Could you check a few things on this model? Use its own coordinates, in mm. Face numbers are marked on the shaded views. A direction names the side the tool comes from. Give positions to 0.01 mm unless a question says otherwise; leave off trailing zeros. Order: outer loops, then holes, each group sorted by start corner. A loop starts at its lowest first (then second) coordinate and runs counter-clockwise, first axis right, second up. Notation, with made-up numbers: (79.5, 75) - (134.5, 75) arc R15 ccw to (134.5, 93) - close; hole circle Ø7 at (-35.5, 80.5). An arc over 180 degrees is marked (long way). One line per question, with ' | ' between items. Start each with the question number.
1. Imagine slicing it at A-A (x = 38). Please give me the cut outline in (y, z), and give its area (3 significant figures).
2. Imagine slicing it at C-C (y = 0). Please give me the cut outline in (x, z), and give its area (3 significant figures).
3. Imagine slicing it at B-B (y = 20.5). Please give me the cut outline in (x, z).
4. Which directions (+Z, -Z, +X, -X, +Y, -Y) give clear straight access to the entire face, cutting with the end or side of a thin tool? Please do the marked faces 3 and 4.
5. Imagine slicing it at D-D (z = 12). Please give me the cut outline in (x, y), and give its area (3 significant figures).
6. If we mould it in two halves opening along Y, with no side actions, what happens to the marked faces 1 and 2? For each: released by +Y, released by -Y, zero draft, split by the parting line, or undercut.
7. I need wall thicknesses on probe 1 along Y at (x, z) = (38, 11.25); probe 2 along Y at (x, z) = (35, 27); probe 3 along Z at (x, y) = (29.5, -25). Which ranges of each line are inside material? Lowest first, please. Write a range as from..to.
8. For P1, Ø2, axis at x = 44, y = -12.5, coming from the +Z side; P2, Ø7, axis at x = 36.5, y = -20, coming from the +Z side; P3, Ø1.5, axis at y = -26, z = 10, coming from the +X side, each with a flat end and sliding along its axis, tell me the tip position at first contact or that it passes through.
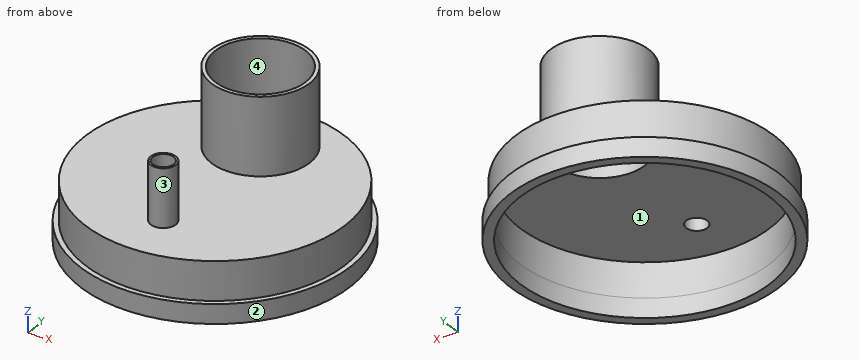
Autodesk Inventor part; units mm, degrees
ref_plane "YZ Plane" through (0, 0, 0) normal (1, 0, 0) x (0, 1, 0)
ref_plane "XZ Plane" through (0, 0, 0) normal (0, 1, 0) x (-1, 0, 0)
ref_plane "XY Plane" through (0, 0, 0) normal (0, 0, 1) x (1, 0, 0)
ref_plane "Plano de trabalho1" through (12.8418, -28.4792, 0) normal (0, 0, 1) x (0.6621, 0.7495, 0)
sketch "Esboço1" plane through (12.8418, -28.4792, 0) normal (0, 0, 1) x (0.6621, 0.7495, 0)
  circle A0 centre (38, 0) radius 32.5
  circle A1 centre (38, 0) radius 35
  point P0 (12.8418, 28.4792)
  dimension "d0" = 70
extrude "Extrusão1" add sketch "Esboço1" along normal blind 5
sketch "Esboço2" plane through (38, 0, 5) normal (0, 0, 1) x (1, 0, 0)
  circle A0 centre (0, 0) radius 34.6774
  circle A1 centre (0, 0) radius 32.5
  circle A2 centre (0, 0) radius 33.6774
  point P0 (-38, 0)
  dimension "d3" = 1
extrude "Extrusão2" add sketch "Esboço2" along normal blind 10 contours A2
sketch "Esboço3" plane through (38, 0, 15) normal (0, 0, 1) x (1, 0, 0)
  circle A0 centre (0, 0) radius 32.5
  point P0 (-38, 0)
extrude "Extrusão3" add sketch "Esboço3" against normal blind 1
sketch "Esboço4" plane through (38, 0, 15) normal (0, 0, 1) x (1, 0, 0)
  circle A0 centre (0, 0) radius 33.6774
  circle A1 centre (0, 17.5016) radius 12.75
  circle A2 centre (0, 17.5016) radius 11.75
  point P0 (-38, 0)
  dimension "d8" = 25.5
  dimension "d9" = 1
extrude "Extrusão4" add sketch "Esboço4" along normal blind 20 contours A1
sketch "Esboço5" plane through (38, 0, 15) normal (0, 0, 1) x (1, 0, 0)
  circle A0 centre (0, 0) radius 33.6774
  circle A1 centre (0, 17.5016) radius 12.75
  circle A2 centre (0, -20) radius 3.25
  circle A3 centre (0, -20) radius 2.75
  point P0 (-38, 0)
  dimension "d12" = 6.5
  dimension "d14" = 0.5
  dimension "d15" = 20
extrude "Extrusão5" add sketch "Esboço5" along normal blind 15 contours A2
sketch "Esboço6" plane through (38, 0, 15) normal (0, 0, 1) x (1, 0, 0)
  circle A0 centre (0, -20) radius 2.75
  circle A1 centre (0, 17.5016) radius 11.75
  point P0 (-38, 0)
extrude "Extrusão6" cut sketch "Esboço6" against normal blind 15
properties part number "Tampa de Entrada"
Results found:
1) outline: (-35, 0) - (-32.5, 0) - (-32.5, 14) - (-22.75, 14) - (-22.75, 30) - (-23.25, 30) - (-23.25, 15) - (-33.68, 15) - (-33.68, 5) - (-35, 5) - close; (-17.25, 14) - (5.75, 14) - (5.75, 35) - (4.75, 35) - (4.75, 15) - (-16.75, 15) - (-16.75, 30) - (-17.25, 30) - close; (29.25, 14) - (32.5, 14) - (32.5, 0) - (35, 0) - (35, 5) - (33.68, 5) - (33.68, 15) - (30.25, 15) - (30.25, 35) - (29.25, 35) - close | area: 140 mm2
2) outline: (3, 0) - (5.5, 0) - (5.5, 14) - (70.5, 14) - (70.5, 0) - (73, 0) - (73, 5) - (71.68, 5) - (71.68, 15) - (4.32, 15) - (4.32, 5) - (3, 5) - close | area: 114 mm2
3) outline: (9.63, 0) - (12.78, 0) - (12.78, 14) - (26.64, 14) - (26.64, 35) - (25.61, 35) - (25.61, 15) - (11.28, 15) - (11.28, 5) - (9.63, 5) - close; (49.36, 14) - (63.22, 14) - (63.22, 0) - (66.37, 0) - (66.37, 5) - (64.72, 5) - (64.72, 15) - (50.39, 15) - (50.39, 35) - (49.36, 35) - close
4) face 3: +Z | face 4: +Z, -Z
5) outline: circle Ø67.35 at (38, 0); hole circle Ø65 at (38, 0) | area: 245 mm2
6) face 1: undercut | face 2: split by the parting line
7) probe 1: y = -33.68..-32.5, 32.5..33.68 | probe 2: y = -21.25..-18.75, 5.11..6.14, 28.86..29.89 | probe 3: z = 14..15
8) P1: stops at z = 15 | P2: stops at z = 30 | P3: stops at x = 60.28
